from build123d import *

# Parameters (mm, degrees)
RESSALTO_EXTRUS_O1_DEPTH = 6.5
ESBO_O2_R                = 14.95
CORTE_EXTRUS_O1_DEPTH    = 9
ESBO_O3_R                = 2.5
CORTE_EXTRUS_O2_DEPTH    = 13
FILETE1_R                = 10
ESBO_O4_R                = 2
CORTE_EXTRUS_O3_DEPTH    = 10
ESBO_O6_R                = 2
CORTE_EXTRUS_O4_DEPTH    = 10
ESBO_O7_R                = 1.5
CORTE_EXTRUS_O5_DEPTH    = 10
FILETE2_R                = 2.5


with BuildPart() as part:
    # Esboço1 → Ressalto-extrusão1 (new, symmetric)
    with BuildSketch(Plane.XY):
        Polygon((32.742040246, 55), (-22.781745931, 55), (-44.375431078, 33.406314852), (-44.375431078, -33.406314852), (-22.781745931, -55), (32.742040246, -55), (32.742040246, -49), (72.742040246, -49), (72.742040246, -43), (32.742040246, -43), (32.742040246, 4), (72.742040246, 4), (72.742040246, 10), (32.742040246, 10), align=None)
    extrude(amount=RESSALTO_EXTRUS_O1_DEPTH, both=True)

    # Esboço2 → Corte-extrusão1 (cut)
    with BuildSketch(Plane.XY.offset(6.5)):
        with Locations((-20, 0)):
            Circle(ESBO_O2_R)
    extrude(amount=-CORTE_EXTRUS_O1_DEPTH, mode=Mode.SUBTRACT)

    # Esboço3 → Corte-extrusão2 (cut)
    with BuildSketch(Plane.XY.offset(6.5)):
        with Locations((8, 22.5)):
            Circle(ESBO_O3_R)
        Polygon((-12.281745931, -55), (32.742040246, -49), (32.742040246, -55), align=None)
        Polygon((32.742040246, 55), (-12.281745931, 55), (32.742040246, 20), align=None)
    extrude(amount=-CORTE_EXTRUS_O2_DEPTH, mode=Mode.SUBTRACT)

    # Filete1
    filete1_edges = [part.edges().sort_by_distance(p)[0] for p in [
        (-22.781745931, -55, 0),
    ]]
    fillet(filete1_edges, radius=FILETE1_R)

    # Esboço4 → Corte-extrusão3 (cut)
    with BuildSketch(Plane(origin=(0, 0, -6.5), x_dir=(-1, 0, 0), z_dir=(0, 0, -1))):
        with Locations((36.375431078, 8.406314852)):
            Circle(ESBO_O4_R)
        with Locations((12.955431078, -16.593685148)):
            Circle(ESBO_O4_R)
        with Locations((22.375431078, -27.593685148)):
            Circle(ESBO_O4_R)
    extrude(amount=-CORTE_EXTRUS_O3_DEPTH, mode=Mode.SUBTRACT)

    # Esboço6 → Corte-extrusão4 (cut)
    with BuildSketch(Plane(origin=(0, 10, 0), x_dir=(1, 0, 0), z_dir=(0, 1, 0))):
        with Locations(Location((42.742040246, -0.001621735, 0), (0, 0, 270))):
            Circle(ESBO_O6_R)
        with Locations(Location((62.742040246, -0.001621735, 0), (0, 0, 270))):
            Circle(ESBO_O6_R)
    extrude(amount=-CORTE_EXTRUS_O4_DEPTH, mode=Mode.SUBTRACT)

    # Esboço7 → Corte-extrusão5 (cut)
    with BuildSketch(Plane.XZ.offset(49)):
        with Locations(Location((37.742040246, 0, 0), (0, 0, 270))):
            Circle(ESBO_O7_R)
        with Locations(Location((52.742040246, 0, 0), (0, 0, 270))):
            Circle(ESBO_O7_R)
        with Locations(Location((67.742040246, 0, 0), (0, 0, 270))):
            Circle(ESBO_O7_R)
    extrude(amount=-CORTE_EXTRUS_O5_DEPTH, mode=Mode.SUBTRACT)

    # Filete2
    filete2_edges = [part.edges().sort_by_distance(p)[0] for p in [
        (32.742040246, 10, 0),
        (72.742040246, 10, 0),
        (72.742040246, 4, 0),
        (32.742040246, 4, 0),
        (32.742040246, -43, 0),
        (72.742040246, -43, 0),
        (72.742040246, -49, 0),
        (32.742040246, 20, 0),
    ]]
    fillet(filete2_edges, radius=FILETE2_R)


solid = part.part
Geometry check sheet. Reference: the model listing, model coordinates, mm. A direction names the side the tool comes from. Round coordinates to 2 decimals unless told otherwise and drop trailing zeros. Write each loop counter-clockwise with the first axis right and the second up, starting at its lowest first coordinate (ties: lowest second). Pieces come first, ordered by that corner, then holes.
Item 1: Access from +Z, -Z, +X, -X, +Y, -Y to the whole of each face (thin tool, end or side, straight path). Record for faces 5 (the face through (51, -49, 0)), 6 (the face through (-20, 0, -2.5)), 7 (the face through (-22, -28, 3.5)), 8 (the face through (51.28, -46.04, 0.33)), 9 (the face through (52, 4, 0)).
Determined:
face 5: +Z, -Z, +X, -Y
face 6: +Z
face 7: -Z
face 8: -Y
face 9: +Z, -Z, +X
Item 2: Mould release check, pull along Y, two halves, no side actions. Record for faces 1 (the face through (-14.803, -17.36, -1.57)), 2 (the face through (9.34, 24.61, 0.09)), 3 (the face through (-16, -55, 0)), 4 (the face through (-33.43, 44.35, 0.09)): +Y half, -Y half, draft (parallel to the pull), parting line (faces both ways), or undercut.
Determined:
face 1: undercut
face 2: undercut
face 3: -Y half
face 4: +Y half
Item 3: Material ranges on line 1 along Y through (x, z) = (46, 4); line 2 along X through (y, z) = (-44.15, 0); line 3 along X through (y, z) = (-22.5, -4.75), recorded low to high.
Determined:
line 1: y = -49 to -43, 4 to 10
line 2: x = -33.63 to 36.24, 39.24 to 51.24, 54.24 to 66.24, 69.24 to 72.35
line 3: x = -44.38 to 32.74
Item 4: Section check C-C (z = 0). Give the number of separate pieces and of enclosed holes in the cut face, plus the area to 3 significant figures.
Determined:
separate pieces: 6
enclosed holes: 5
area: 6,710 mm2
Item 5: Section check B-B (x = 8). Record the boundary of the cut face in (y, z), plus the area to 3 significant figures.
Determined:
outline: (-52.3, -6.5) - (20, -6.5) - (20, 6.5) - (-52.3, 6.5) - close; (25, -6.5) - (39.23, -6.5) - (39.23, 6.5) - (25, 6.5) - close
area: 1,120 mm2
Item 6: Section check A-A (y = 22.5). Record the boundary of the cut face in (x, z).
Determined:
outline: (-44.38, -6.5) - (5.5, -6.5) - (5.5, 6.5) - (-44.38, 6.5) - close; (10.5, -6.5) - (29.53, -6.5) - (29.53, 6.5) - (10.5, 6.5) - close
Item 7: Section check D-D (x = -8). Record the boundary of the cut face in (y, z), plus the area to 3 significant figures.
Determined:
outline: (-54.43, -6.5) - (51.67, -6.5) - (51.67, 6.5) - (8.92, 6.5) - (8.92, -2.5) - (-8.92, -2.5) - (-8.92, 6.5) - (-54.43, 6.5) - close
area: 1,220 mm2
Item 8: Go/stop test with flat-tipped pins: pin 1 Ø4 at (x, z) = (67.74, 0) entering from +Y; pin 2 Ø1.5 at (x, z) = (54, -4.5) entering from -Y; pin 3 Ø4 at (x, z) = (-24, -3) entering from -Y. Record where each tip stops, or that it passes through.
Determined:
pin 1: stops at y = 10
pin 2: stops at y = -49
pin 3: stops at y = -54.42
